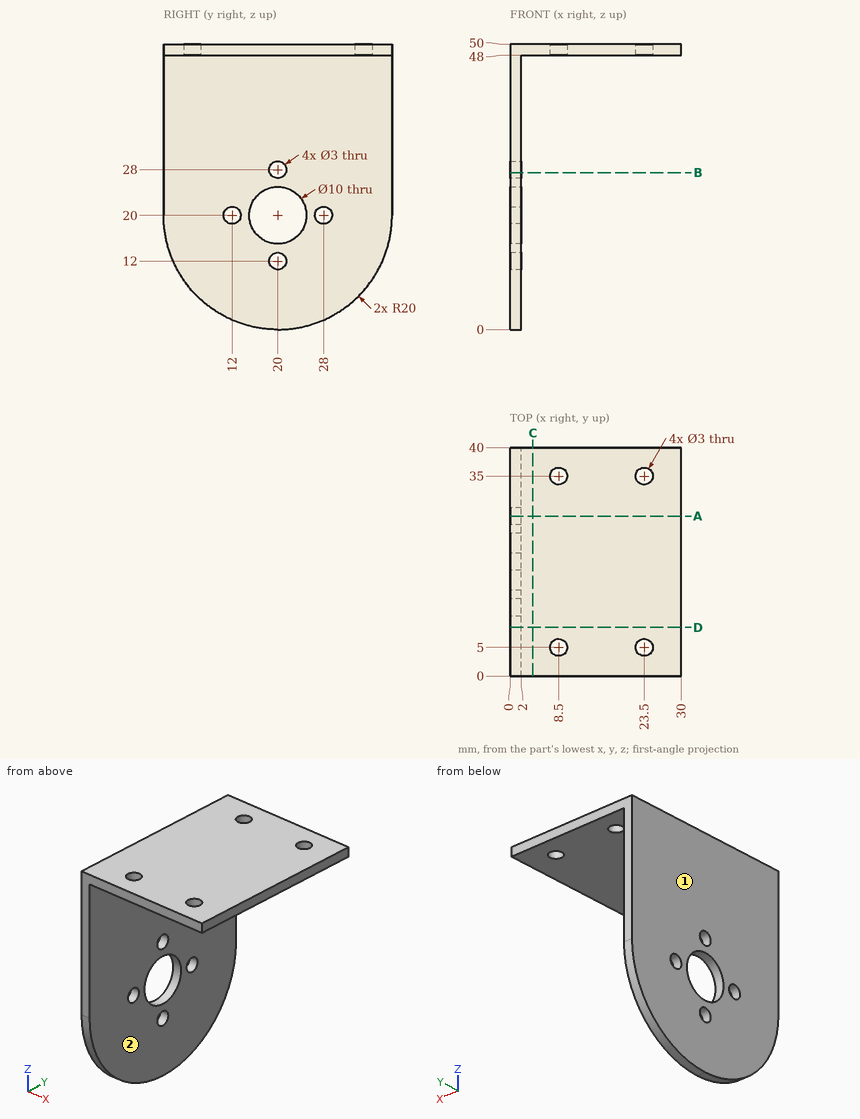
The figure shows three views and two pictorial views of one solid part (mm, origin at its lowest corner). Answer the questions. A direction names the side the tool comes from. Give positions to 0.01 mm unless a question says otherwise; leave off trailing zeros. Loops run counter-clockwise (first coordinate to the right, second up) from the corner with the lowest first, then second, coordinate; pieces in that order, holes last. Notation, with made-up numbers: (85.5, 61) -> (117.5, 61) arc R31 ccw to (117.5, 87) -> close; hole circle Ø1 at (6, 80.5). An arc over 180 degrees is marked (long way). Use a Markdown table: item, result. Add a question column.
1. For the marked faces 1 and 2, determine the directions among +Z, -Z, +X, -X, +Y, -Y from which every point of the face is accessible in a straight line to the end or side of a thin tool.
2. Find the intervals of material crossed by probe 1 along Z at (x, y) = (7, 18.5); probe 2 along X at (y, z) = (13.5, 9.5); probe 3 along Y at (x, z) = (23, 49), in increasing order.
3. Section A-A on y = 28 is taken. Determine the outline of the cut face in (x, z), and give its area (3 significant figures).
4. Section C-C on x = 4 is taken. Determine the outline of the cut face in (y, z).
5. Section B-B on z = 27.5 is taken. Determine the outline of the cut face in (x, y).
6. Flat-ended cylindrical pins translate along their axes: pin 1 Ø5 at (y, z) = (33, 18.5) entering from +X; pin 2 Ø3.5 at (x, y) = (23.5, 5) entering from -Z. Find the tip coordinate at first contact, or state that the pin passes through.
7. Section D-D on y = 8.5 is taken. Determine the outline of the cut face in (x, z).
Results below:
| question | item | result |
|---|---|---|
| 1 | face 1 | +Z, -Z, -X, +Y, -Y |
| 1 | face 2 | -Z, +X, +Y, -Y |
| 2 | probe 1 | z = 48 to 50 |
| 2 | probe 2 | x = 0 to 2 |
| 2 | probe 3 | y = 0 to 3.59, 6.41 to 33.59, 36.41 to 40 |
| 3 | outline | (0, 1.67) -> (2, 1.67) -> (2, 18.5) -> (0, 18.5) -> close; (0, 21.5) -> (2, 21.5) -> (2, 48) -> (30, 48) -> (30, 50) -> (0, 50) -> close |
| 3 | area | 147 mm^2 |
| 4 | outline | (0, 48) -> (40, 48) -> (40, 50) -> (0, 50) -> close |
| 5 | outline | (0, 0) -> (2, 0) -> (2, 18.59) -> (0, 18.59) -> close; (0, 21.41) -> (2, 21.41) -> (2, 40) -> (0, 40) -> close |
| 6 | pin 1 | stops at x = 2 |
| 6 | pin 2 | stops at z = 48 |
| 7 | outline | (0, 3.64) -> (2, 3.64) -> (2, 48) -> (30, 48) -> (30, 50) -> (0, 50) -> close |
